Drawing for the job (mm, zero at the part's lowest x, y, z). Coordinates: 2 decimals unless noted, no trailing zeros. Write each loop counter-clockwise with the first axis right and the second up, starting at its lowest first coordinate (ties: lowest second). Pieces come first, ordered by that corner, then holes. Notation, with made-up numbers: (34, -4.5) - (53, -4.5) arc R26 cw to (53, 31.5) - close; hole circle Ø7 at (16.5, 83.5). An arc over 180 degrees is marked (long way). Write each question's results on one line, items separated by ' | '.
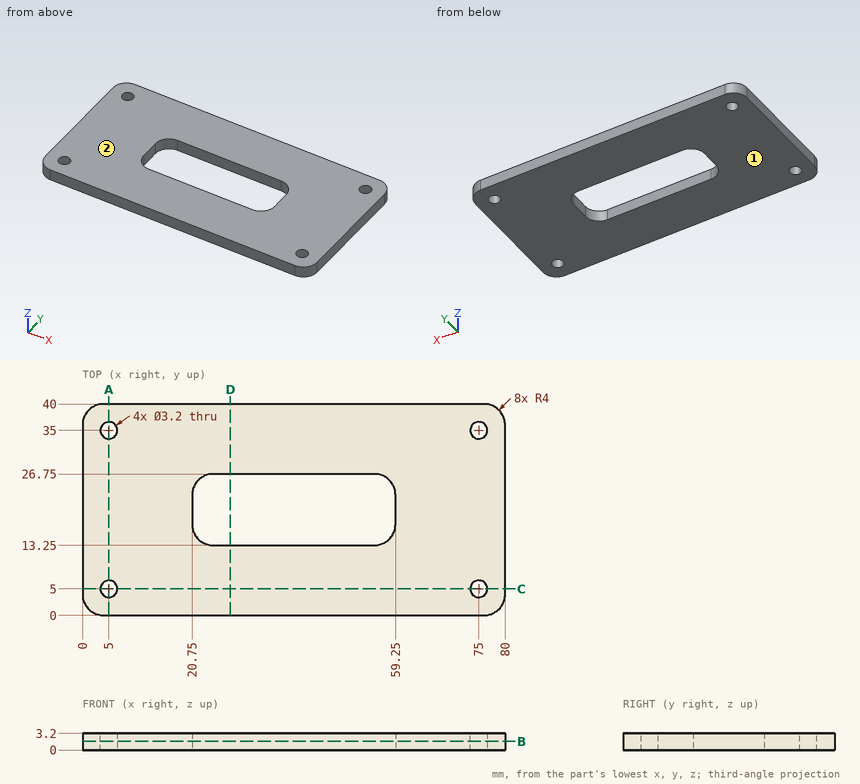
(1) Wall check: line 1 (Y direction, x = 75, z = 2.05); line 2 (X direction, y = 22.5, z = 1.75); line 3 (Y direction, x = 31, z = 2.1). Give the ranges that are in metal, low to high. Write a range as from..to.
Return value:
line 1: y = 0..3.4, 6.6..33.4, 36.6..40 | line 2: x = 0..20.75, 59.25..80 | line 3: y = 0..13.25, 26.75..40
(2) Saw through at D-D on x = 28. Write the cut outline in (y, z), then the cut area to 3 significant figures.
Return value:
outline: (0, 0) - (13.25, 0) - (13.25, 3.2) - (0, 3.2) - close; (26.75, 0) - (40, 0) - (40, 3.2) - (26.75, 3.2) - close | area: 84.8 mm^2
(3) Saw through at B-B on z = 1.7. Write the cut outline in (x, y).
Return value:
outline: (0, 4) arc R4 ccw to (4, 0) - (76, 0) arc R4 ccw to (80, 4) - (80, 36) arc R4 ccw to (76, 40) - (4, 40) arc R4 ccw to (0, 36) - close; hole circle Ø3.2 at (5, 5); hole circle Ø3.2 at (5, 35); hole (20.75, 17.25) arc R4 ccw to (24.75, 13.25) - (55.25, 13.25) arc R4 ccw to (59.25, 17.25) - (59.25, 22.75) arc R4 ccw to (55.25, 26.75) - (24.75, 26.75) arc R4 ccw to (20.75, 22.75) - close; hole circle Ø3.2 at (75, 5); hole circle Ø3.2 at (75, 35)
(4) Flat gauge pin, fed straight in: P1, Ø3, axis at x = 5, y = 5, coming from the -Z side. Where does the tip first touch, or does it go through?
Return value:
P1: passes through
(5) Saw through at C-C on y = 5. Write the cut outline in (x, z).
Return value:
outline: (0, 0) - (3.4, 0) - (3.4, 3.2) - (0, 3.2) - close; (6.6, 0) - (73.4, 0) - (73.4, 3.2) - (6.6, 3.2) - close; (76.6, 0) - (80, 0) - (80, 3.2) - (76.6, 3.2) - close
(6) Two-plate mould, pull along Z, no slides. Class the marked faces 1 and 2: released by +Z, released by -Z, zero draft, split by the parting line, or undercut.
Return value:
face 1: released by -Z | face 2: released by +Z
(7) Saw through at A-A on x = 5. Write the cut outline in (y, z).
Return value:
outline: (0, 0) - (3.4, 0) - (3.4, 3.2) - (0, 3.2) - close; (6.6, 0) - (33.4, 0) - (33.4, 3.2) - (6.6, 3.2) - close; (36.6, 0) - (40, 0) - (40, 3.2) - (36.6, 3.2) - close
